Model file for the job. Use its own axes, mm. A direction names the side the tool comes from. Coordinates: 2 decimals unless noted, no trailing zeros. Write each loop counter-clockwise with the first axis right and the second up, starting at its lowest first coordinate (ties: lowest second). Pieces come first, ordered by that corner, then holes. Notation, with made-up numbers: M 57,-15.5 L 116,-15.5 A19 cw 116,8.5 Z; hole C 55.5,-25.75 d11. An arc over 180 degrees is marked long. Put each result on its own line as item: value. Start each with the question number.
Q1. Cut at A-A (y = -0.65). Write the cut outline in (x, z).
Q2. Cut at B-B (x = 21). Write the cut outline in (y, z).
Q3. Drop flat-ended pins along their axis: pin 1 (0.8 mm diameter, centred on x = 25.5, y = -0.5, fed in from +Z); pin 2 (0.8 mm diameter, centred on x = 18, y = -0.5, fed in from -Z); pin 3 (0.8 mm diameter, centred on y = -0.5, z = 4.5, fed in from +X). Give the stop position or say it passes through.
Q4. Which spindle directions (+Z, -Z, +X, -X, +Y, -Y) get a long thin tool onto all of the face, cutting with end or side? Do faces 1 (the flat face through (18, -0.5, 1.95)), 2 (the cylindrical face through (34, -0.49, 8.12)), 3 (the cylindrical face through (2.4, -0.49, 2.38)), 4 (the flat face through (1.95, -0.5, 5.3)). Say none if no direction does.
Q5. Drill centre lines: line 1 along Y through (x, z) = (10.5, 1); line 2 along Z through (x, y) = (16, -0.8); line 3 along X through (y, z) = (-0.8, 3). Where is each one in solid material? Low to high.
Autodesk Inventor part; units mm, degrees
ref_plane "YZ Plane" through (0, 0, 0) normal (1, 0, 0) x (0, 1, 0)
ref_plane "XZ Plane" through (0, 0, 0) normal (0, 1, 0) x (-1, 0, 0)
ref_plane "XY Plane" through (0, 0, 0) normal (0, 0, 1) x (1, 0, 0)
sketch "Эскиз1" plane through (0, 0, 0) normal (0, 1, 0) x (-1, 0, 0)
  line L0 (-3.45, 1.95) -> (-32.95, 1.95)
  line L1 (-34.45, 3.45) -> (-34.45, 7.05)
  line L2 (-32.95, 8.55) -> (-3.45, 8.55)
  line L3 (-1.95, 7.05) -> (-1.95, 3.45)
  line L4 (-1.5, 0) -> (-34.9, 0)
  line L5 (-36.4, 1.5) -> (-36.4, 9)
  line L6 (-34.9, 10.5) -> (-1.5, 10.5)
  line L7 (0, 9) -> (0, 1.5)
  arc A0 (-3.45, 1.95) -> (-1.95, 3.45) centre (-3.45, 3.45) ccw
  arc A1 (-1.95, 7.05) -> (-3.45, 8.55) centre (-3.45, 7.05) ccw
  arc A2 (-32.95, 8.55) -> (-34.45, 7.05) centre (-32.95, 7.05) ccw
  arc A3 (-34.45, 3.45) -> (-32.95, 1.95) centre (-32.95, 3.45) ccw
  arc A4 (-36.4, 1.5) -> (-34.9, 0) centre (-34.9, 1.5) ccw
  arc A5 (-34.9, 10.5) -> (-36.4, 9) centre (-34.9, 9) ccw
  arc A6 (0, 9) -> (-1.5, 10.5) centre (-1.5, 9) ccw
  arc A7 (-1.5, 0) -> (0, 1.5) centre (-1.5, 1.5) ccw
  point P0 (0, 0)
  point P1 (-34.45, 1.95)
  point P2 (-1.95, 8.55)
  point P3 (0, 0)
  point P4 (-36.4, 10.5)
  dimension "d6" = 1.5
  dimension "d7" = 1.5
  dimension "d8" = 1.5
  dimension "d9" = 1.5
  dimension "d10" = 1.5
  dimension "d11" = 1.5
  dimension "d12" = 1.5
  dimension "d13" = 1.5
extrude "Выдавливание3" add sketch "Эскиз1" against normal blind 1 contours L0 A3 L1 A2 L2 A1 L3 A0
extrude "Выдавливание4" add sketch "Эскиз1" against normal blind 2 from surface at -1 contours L0 A3 L1 A2 L2 A1 L3 A0 | L4 A4 L5 A5 L6 A6 L7 A7
properties part number "screen3"
Computed values:
1. outline: M 1.95,3.45 A1.5 ccw 3.45,1.95 L 32.95,1.95 A1.5 ccw 34.45,3.45 L 34.45,7.05 A1.5 ccw 32.95,8.55 L 3.45,8.55 A1.5 ccw 1.95,7.05 Z
2. outline: M -3,0 L -1,0 L -1,1.95 L 0,1.95 L 0,8.55 L -1,8.55 L -1,10.5 L -3,10.5 Z
3. pin 1: z = 8.55
3. pin 2: z = 1.95
3. pin 3: x = 34.45
4. face 1: -Z, +X, -X, +Y
4. face 2: +Z, +X, +Y
4. face 3: -Z, -X, +Y
4. face 4: +Z, -Z, -X, +Y
5. line 1: -3 to -1
5. line 2: 1.95 to 8.55
5. line 3: 2.02 to 34.38
